Input: dimensioned drawing with shaded views. Units: mm. Origin: part minimum x, y, z. A direction names the side the tool comes from. Coordinates: 2 decimals unless noted, no trailing zeros. Order: outer loops, then holes, each group sorted by start corner. A loop starts at its lowest first (then second) coordinate and runs counter-clockwise, first axis right, second up. Notation, with made-up numbers: (27.25, 25) -> (71.25, 25) arc R29 cw to (71.25, 61) -> close; hole circle Ø5 at (-24.5, 86.25). An arc over 180 degrees is marked (long way). Write item = value, one per line. Start each with the question number.
Item 1: Section query C-C (x = 45.5). Output: boundary loops of the cut face in (y, z).
Item 2: Section query D-D (z = 9). Output: boundary loops of the cut face in (x, y), then the cut area to 3 significant figures.
Item 3: Section query B-B (y = 9). Output: boundary loops of the cut face in (x, z).
Item 4: Contact query for flat-ended pins moving along their axis: pin 1 (8 mm diameter, centred on x = 41.5, y = 40, fed in from -Z); pin 2 (4 mm diameter, centred on y = 7, z = 10, fed in from +X); pin 3 (13 mm diameter, centred on y = 35, z = 10, fed in from -X). Output: stop coordinate, or through.
Item 5: Mould query, pull axis X, two halves, no side actions, for the marked faces 5, 6 and 7. Classes: released by +X, released by -X, zero draft, split by the parting line, or undercut.
Item 6: Ray query, line 1 along X through (y, z) = (5.65, 0.7); line 2 along Z through (x, y) = (8, 8); line 3 along Y through (x, z) = (24, 22). Return the intervals inside material, ascending. Write a range as [from, to].
Item 7: Set-up query: the marked faces 1, 2, 3 and 4. Return all of +Z, -Z, +X, -X, +Y, -Y with unobstructed straight access to the full face (end or side cutting, diameter ignored); none if empty.
Item 8: Section query A-A (x = 26.5). Output: boundary loops of the cut face in (y, z), then the cut area to 4 significant figures.
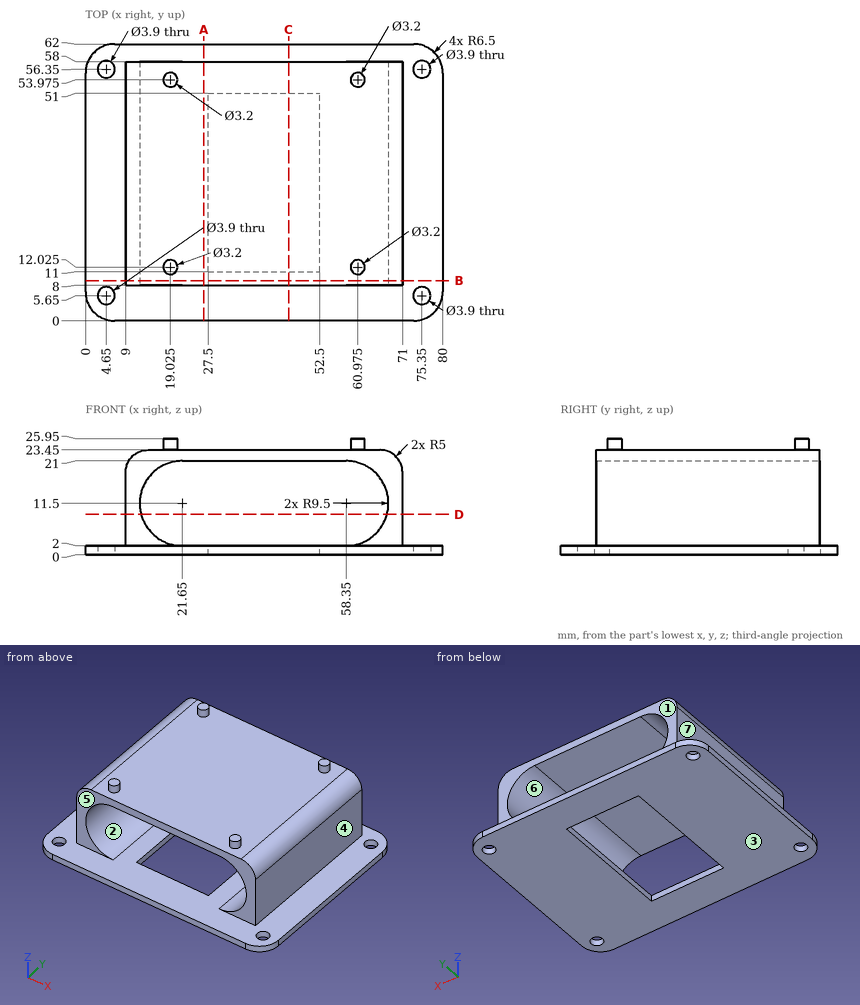
Computed:
q1.outline = (0, 0) -> (11, 0) -> (11, 2) -> (0, 2) -> close; (8, 21) -> (58, 21) -> (58, 23.45) -> (8, 23.45) -> close; (51, 0) -> (62, 0) -> (62, 2) -> (51, 2) -> close
q2.outline = (9, 8) -> (12.48, 8) -> (12.48, 58) -> (9, 58) -> close; (67.52, 8) -> (71, 8) -> (71, 58) -> (67.52, 58) -> close
q2.area = 348 mm^2
q3.outline = (0, 0) -> (80, 0) -> (80, 2) -> (71, 2) -> (71, 18.45) arc R5 ccw to (66, 23.45) -> (14, 23.45) arc R5 ccw to (9, 18.45) -> (9, 2) -> (0, 2) -> close; hole (21.65, 2) -> (58.35, 2) arc R9.5 ccw to (58.35, 21) -> (21.65, 21) arc R9.5 ccw to start
q4.pin_1 = 21
q4.pin_2 = 71
q4.pin_3 = 9
q5.face_5 = zero draft
q5.face_6 = undercut
q5.face_7 = released by -X
q6.line_1 = [0.06, 2.7], [6.6, 73.4], [77.3, 79.94]
q6.line_2 = [0, 2]
q6.line_3 = [8, 58]
q7.face_1 = +Z, +X, -X, +Y
q7.face_2 = +Y, -Y
q7.face_3 = -Z, +X, -X, +Y, -Y
q7.face_4 = +Z, +X, +Y, -Y
q8.outline = (0, 0) -> (62, 0) -> (62, 2) -> (0, 2) -> close; (8, 21) -> (58, 21) -> (58, 23.45) -> (8, 23.45) -> close
q8.area = 246.5 mm^2
